For this review, take the finished solid that the model builds, in its own axes (mm). Face numbers are marked on the shaded views. Give positions to 0.01 mm unless a question says otherwise; leave off trailing zeros. Loops run counter-clockwise (first coordinate to the right, second up) from the corner with the lowest first, then second, coordinate; pieces in that order, holes last. Notation, with made-up numbers: (9.5, 25.25) - (26.5, 25.25) arc R9 cw to (26.5, 31.25) - close; hole circle Ø1 at (39.5, -19). An arc over 180 degrees is marked (long way). Use CSV: the item, a comma, the result in double quotes. Start each with the question number.
1. Mouldability with a two-part tool opening along Y and no side actions: class the marked faces 1, 2 and 3 as pulls with the +Y half, pulls with the -Y half, needs draft (parallel to the pull), parting line crosses it, or undercut.
2. Take a section at A-A on y = 0. Give the boundary of the cut face in (x, z).
3. For pin 1 (1.5 mm diameter, centred on x = 13, z = 2.5, fed in from +Y); pin 2 (10 mm diameter, centred on x = -13.5, y = -12, fed in from -Z); pin 3 (2 mm diameter, centred on x = 8.5, z = 2.5, fed in from -Y); pin 4 (1 mm diameter, centred on x = -7.5, z = 2.5, fed in from +Y), all flat-tipped, find the tip position at first contact; note any pin that passes through.
4. Take a section at D-D on x = 4.5. Give the boundary of the cut face in (y, z).
5. Wall thickness on line 1 (Y direction, x = 0, z = 7.6); line 2 (Y direction, x = 0, z = 4.3); line 3 (Z direction, x = 2, y = 5): over which ranges is each line inside the solid? List them lowest first.
6. Take a section at B-B on z = 6.75. Give the boundary of the cut face in (x, y).
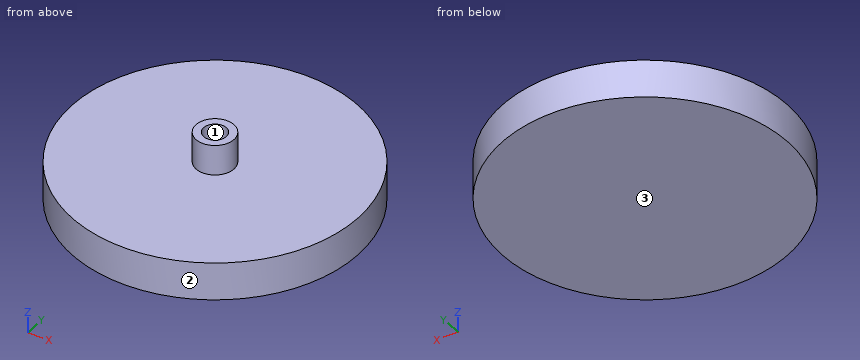
```python
from build123d import *

# Parameters (mm, degrees)
F0_R     = 18.85
F0_R_2   = 2.5
F0_R_3   = 1.5
F1_DEPTH = 5
F2_DEPTH = 9
F3_DEPTH = 3


with BuildPart() as f1:
    # F0 (on Top) → F1 (new body)
    with BuildSketch(Plane.XY):
        Circle(F0_R)
        Circle(F0_R_2, mode=Mode.SUBTRACT)
        Circle(F0_R_2)
        Circle(F0_R_3, mode=Mode.SUBTRACT)
    extrude(amount=F1_DEPTH)

    # F0 (on Top) → F2 (join)
    with BuildSketch(Plane.XY):
        Circle(F0_R_2)
        Circle(F0_R_3, mode=Mode.SUBTRACT)
    extrude(amount=F2_DEPTH)

    # F0 (on Top) → F3 (join)
    with BuildSketch(Plane.XY):
        Circle(F0_R)
        Circle(F0_R_2, mode=Mode.SUBTRACT)
        Circle(F0_R_3)
    extrude(amount=F3_DEPTH)


solid = f1.part
```
Check result:
1,face 1,"undercut"
1,face 2,"parting line crosses it"
1,face 3,"needs draft"
2,outline,"(-18.85, 0) - (18.85, 0) - (18.85, 5) - (2.5, 5) - (2.5, 9) - (1.5, 9) - (1.5, 3) - (-1.5, 3) - (-1.5, 9) - (-2.5, 9) - (-2.5, 5) - (-18.85, 5) - close"
3,pin 1,"stops at y = 14.33"
3,pin 2,"stops at z = 0"
3,pin 3,"stops at y = -17.29"
3,pin 4,"stops at y = 17.5"
4,outline,"(-18.3, 0) - (18.3, 0) - (18.3, 5) - (-18.3, 5) - close"
5,line 1,"y = -2.5 to -1.5, 1.5 to 2.5"
5,line 2,"y = -18.85 to -1.5, 1.5 to 18.85"
5,line 3,"z = 0 to 5"
6,outline,"circle Ø5 at (0, 0); hole circle Ø3 at (0, 0)"
